Here's how the part is built. I have some questions about the finished solid (model axes, mm). A direction names the side the tool comes from. Round coordinates to 2 decimals unless told otherwise and drop trailing zeros. Write each loop counter-clockwise with the first axis right and the second up, starting at its lowest first coordinate (ties: lowest second). Pieces come first, ordered by that corner, then holes. Notation, with made-up numbers: (86, 43) -> (120, 43) arc R22 ccw to (120, 79) -> close; hole circle Ø6 at (89.25, -37). An arc over 180 degrees is marked (long way). Answer in a Markdown table with one row per item. Add a question column.
Autodesk Inventor part; units mm, degrees
ref_plane "YZ Plane" through (0, 0, 0) normal (1, 0, 0) x (0, 1, 0)
ref_plane "XZ Plane" through (0, 0, 0) normal (0, 1, 0) x (-1, 0, 0)
ref_plane "XY Plane" through (0, 0, 0) normal (0, 0, 1) x (1, 0, 0)
sketch "Sketch1" plane through (0, 0, 0) normal (0, 1, 0) x (-1, 0, 0)
  circle A0 centre (0, 0) radius 450
  circle A1 centre (0, 0) radius 470
  line L0 (470, 0) -> (450, 0)
  line L1 (-470, 0) -> (-450, 0)
  line L2 (0, 0) -> (-389.7114, 225) construction
  line L3 (0, 450) -> (0, 0) construction
  line L4 (0, 470) -> (0, 450)
  line L5 (-389.7114, 225) -> (-407.0319, 235)
  line L6 (-389.6755, 233.0622) -> (-400.0678, 239.0622)
  line L7 (-400.0678, 239.0622) -> (-401.3614, 231.7261)
  line L8 (-389.6755, 233.0622) -> (-395.382, 228.2739)
  line L9 (-398.3717, 230) -> (-394.8717, 236.0622) construction
  line L10 (7, 454) -> (0, 456.5478)
  line L11 (7, 454) -> (7, 466)
  line L12 (7, 466) -> (0, 463.4522)
  line L13 (396.6755, 220.9378) -> (395.382, 228.2739)
  line L14 (396.6755, 220.9378) -> (407.0678, 226.9378)
  line L15 (407.0678, 226.9378) -> (401.3614, 231.7261)
  line L16 (389.6755, -233.0622) -> (395.382, -228.2739)
  line L17 (389.6755, -233.0622) -> (400.0678, -239.0622)
  line L18 (400.0678, -239.0622) -> (401.3614, -231.7261)
  line L19 (-7, -454) -> (0, -456.5478)
  line L20 (-7, -454) -> (-7, -466)
  line L21 (-7, -466) -> (0, -463.4522)
  line L22 (-396.6755, -220.9378) -> (-395.382, -228.2739)
  line L23 (-396.6755, -220.9378) -> (-407.0678, -226.9378)
  line L24 (-407.0678, -226.9378) -> (-401.3614, -231.7261)
  line L25 (-363.084, 285.1192) -> (-343.7989, 308.0994)
  line L26 (-343.7989, 308.0994) -> (-341.3477, 306.0423)
  line L27 (-341.3477, 306.0423) -> (-360.6327, 283.0622)
  line L28 (-360.6327, 283.0622) -> (-363.084, 285.1192)
  line L29 (-363.084, 285.1192) -> (-341.3477, 306.0423) construction
  line L30 (-343.7989, 308.0994) -> (-360.6327, 283.0622) construction
  circle A2 centre (0, 0) radius 460.0533 construction
  line L31 (-435.6969, 142.6478) -> (-438.7038, 143.7424)
  line L32 (-438.7038, 143.7424) -> (-428.4415, 171.9326)
  line L33 (-425.4346, 170.8379) -> (-435.6969, 142.6478)
  line L34 (-428.4415, 171.9326) -> (-425.4346, 170.8379)
  line L35 (-458.2096, -14.9721) -> (-461.4096, -14.9719)
  line L36 (-461.4096, -14.9719) -> (-461.4077, 15.0281)
  line L37 (-458.2077, 15.0279) -> (-458.2096, -14.9721)
  line L38 (-461.4077, 15.0281) -> (-458.2077, 15.0279)
  line L39 (-425.4554, -170.786) -> (-428.4625, -171.8803)
  line L40 (-428.4625, -171.8803) -> (-438.7214, -143.6889)
  line L41 (-435.7143, -142.5946) -> (-425.4554, -170.786)
  line L42 (-438.7214, -143.6889) -> (-435.7143, -142.5946)
  line L43 (-341.385, -306.0007) -> (-343.8365, -308.0575)
  line L44 (-343.8365, -308.0575) -> (-363.1187, -285.075)
  line L45 (-360.6673, -283.0182) -> (-341.385, -306.0007)
  line L46 (-363.1187, -285.075) -> (-360.6673, -283.0182)
  line L47 (-216.1386, -404.3072) -> (-217.7388, -407.0783)
  line L48 (-217.7388, -407.0783) -> (-243.7186, -392.0768)
  line L49 (-242.1185, -389.3056) -> (-216.1386, -404.3072)
  line L50 (-243.7186, -392.0768) -> (-242.1185, -389.3056)
  line L51 (-64.8227, -453.8482) -> (-65.3785, -456.9996)
  line L52 (-65.3785, -456.9996) -> (-94.9224, -451.7883)
  line L53 (-94.3666, -448.637) -> (-64.8227, -453.8482)
  line L54 (-94.9224, -451.7883) -> (-94.3666, -448.637)
  line L55 (94.3118, -448.6485) -> (94.8673, -451.7999)
  line L56 (94.8673, -451.7999) -> (65.3228, -457.0075)
  line L57 (64.7673, -453.8561) -> (94.3118, -448.6485)
  line L58 (65.3228, -457.0075) -> (64.7673, -453.8561)
  line L59 (242.071, -389.3351) -> (243.6708, -392.1065)
  line L60 (243.6708, -392.1065) -> (217.6891, -407.1049)
  line L61 (216.0893, -404.3335) -> (242.071, -389.3351)
  line L62 (217.6891, -407.1049) -> (216.0893, -404.3335)
  line L63 (360.6327, -283.0622) -> (363.084, -285.1192)
  line L64 (363.084, -285.1192) -> (343.7989, -308.0994)
  line L65 (341.3477, -306.0423) -> (360.6327, -283.0622)
  line L66 (343.7989, -308.0994) -> (341.3477, -306.0423)
  line L67 (435.6969, -142.6478) -> (438.7038, -143.7424)
  line L68 (438.7038, -143.7424) -> (428.4415, -171.9326)
  line L69 (425.4346, -170.8379) -> (435.6969, -142.6478)
  line L70 (428.4415, -171.9326) -> (425.4346, -170.8379)
  line L71 (458.2096, 14.9721) -> (461.4096, 14.9719)
  line L72 (461.4096, 14.9719) -> (461.4077, -15.0281)
  line L73 (458.2077, -15.0279) -> (458.2096, 14.9721)
  line L74 (461.4077, -15.0281) -> (458.2077, -15.0279)
  line L75 (425.4554, 170.786) -> (428.4625, 171.8803)
  line L76 (428.4625, 171.8803) -> (438.7214, 143.6889)
  line L77 (435.7143, 142.5946) -> (425.4554, 170.786)
  line L78 (438.7214, 143.6889) -> (435.7143, 142.5946)
  line L79 (341.385, 306.0007) -> (343.8365, 308.0575)
  line L80 (343.8365, 308.0575) -> (363.1187, 285.075)
  line L81 (360.6673, 283.0182) -> (341.385, 306.0007)
  line L82 (363.1187, 285.075) -> (360.6673, 283.0182)
  line L83 (216.1386, 404.3072) -> (217.7388, 407.0783)
  line L84 (217.7388, 407.0783) -> (243.7186, 392.0768)
  line L85 (242.1185, 389.3056) -> (216.1386, 404.3072)
  line L86 (243.7186, 392.0768) -> (242.1185, 389.3056)
  line L87 (64.8227, 453.8482) -> (65.3785, 456.9996)
  line L88 (65.3785, 456.9996) -> (94.9224, 451.7883)
  line L89 (94.3666, 448.637) -> (64.8227, 453.8482)
  line L90 (94.9224, 451.7883) -> (94.3666, 448.637)
  line L91 (-94.3118, 448.6485) -> (-94.8673, 451.7999)
  line L92 (-94.8673, 451.7999) -> (-65.3228, 457.0075)
  line L93 (-64.7673, 453.8561) -> (-94.3118, 448.6485)
  line L94 (-65.3228, 457.0075) -> (-64.7673, 453.8561)
  line L95 (-242.071, 389.3351) -> (-243.6708, 392.1065)
  line L96 (-243.6708, 392.1065) -> (-217.6891, 407.1049)
  line L97 (-216.0893, 404.3335) -> (-242.071, 389.3351)
  line L98 (-217.6891, 407.1049) -> (-216.0893, 404.3335)
  point P0 (460, 0)
  point P1 (-460, 0)
  point P2 (7, 460)
  point P3 (401.8717, 223.9378)
  point P4 (394.8717, -236.0622)
  point P5 (-7, -460)
  point P6 (-401.8717, -223.9378)
  point P7 (-352.2158, 295.5808)
  point P8 (7, 460)
  point P9 (-361.8584, 284.0907)
  point P10 (-342.5733, 307.0709)
  point P11 (-437.2004, 143.1951)
  point P12 (-426.938, 171.3853)
  point P13 (-459.8096, -14.972)
  point P14 (-459.8077, 15.028)
  point P15 (-426.959, -171.3332)
  point P16 (-437.2178, -143.1418)
  point P17 (-342.6108, -307.0291)
  point P18 (-361.893, -284.0466)
  point P19 (-216.9387, -405.6927)
  point P20 (-242.9185, -390.6912)
  point P21 (-65.1006, -455.4239)
  point P22 (-94.6445, -450.2126)
  point P23 (94.5896, -450.2242)
  point P24 (65.045, -455.4318)
  point P25 (242.8709, -390.7208)
  point P26 (216.8892, -405.7192)
  point P27 (361.8584, -284.0907)
  point P28 (342.5733, -307.0709)
  point P29 (437.2004, -143.1951)
  point P30 (426.938, -171.3853)
  point P31 (459.8096, 14.972)
  point P32 (459.8077, -15.028)
  point P33 (426.959, 171.3332)
  point P34 (437.2178, 143.1418)
  point P35 (342.6108, 307.0291)
  point P36 (361.893, 284.0466)
  point P37 (216.9387, 405.6927)
  point P38 (242.9185, 390.6912)
  point P39 (65.1006, 455.4239)
  point P40 (94.6445, 450.2126)
  point P41 (-94.5896, 450.2242)
  point P42 (-65.045, 455.4318)
  point P43 (-242.8709, 390.7208)
  point P44 (-216.8892, 405.7192)
  dimension "d0" = 900
  dimension "d1" = 940
  dimension "d4" = 60
  dimension "d5" = 7
  dimension "d6" = 70
  dimension "d8" = 12
  dimension "d11" = 360
  dimension "d13" = 3.2
  dimension "d14" = 30
  dimension "d15" = 50
  dimension "d18" = 360
extrude "Extrusion1" add sketch "Sketch1" along normal blind 3 contours A0 L5 L8 L6 L7 A1 L4 | L4 L12 L11 L10
properties part number "D90_CM_CIRCULO"
Item 1: If we section it at D-D on x = 258: Please give me the cut outline in (y, z) (3 decimals).
Item 2: If we mould it in two halves opening along Z, with no side actions, what happens to faces 1 (the cylindrical face through (237.977, 1.479, 405.298)), 2 (the flat face through (353.576, 1.479, 296.448)), 3 (the cylindrical face through (227.85, 1.48, 388.05))? For each: pulls with the +Z half, pulls with the -Z half, needs draft (parallel to the pull), parting line crosses it, or undercut.
Item 3: I need wall thicknesses on line 1 along X through (y, z) = (0.55, 392.5); line 2 along X through (y, z) = (2.65, 289.5); line 3 along Z through (x, y) = (68, 0.5). Which ranges of each line are inside material? Lowest first, please. Write a range as from..to.
Item 4: If we section it at C-C on z = 339.5: Please give me the cut outline in (x, y).
Item 5: If we section it at B-B on y = 2.15: Please give me the cut outline in (x, z).
Item 6: On a 3-axis mill with a long thin cutter (end or side, diameter ignored), from which of +Z, -Z, +X, -X, +Y, -Y can I reach the whole of each face in a straight line? I mean faces 4 (the flat face through (230.86, 1.48, 399.5)), 5 (the flat face through (216, 3, 403)). Say none if no direction works.
Item 7: For P1, Ø1.5, axis at y = 0.5, z = 406, coming from the -X side, with a flat end and sliding along its axis, tell me the tip position at first contact or that it passes through.
Item 8: If we section it at A-A on x = 75: Please give me the cut outline in (y, z).
Results list:
| question | item | result |
|---|---|---|
| 1 | outline | (0, 368.695) -> (3, 368.695) -> (3, 392.856) -> (0, 392.856) -> close |
| 2 | face 1 | pulls with the +Z half |
| 2 | face 2 | undercut |
| 2 | face 3 | pulls with the -Z half |
| 3 | line 1 | 220.1..236.59, 242.99..258.54 |
| 3 | line 2 | 344.51..355.23, 359.41..370.26 |
| 3 | line 3 | 444.83..453.29, 456.54..465.05 |
| 4 | outline | (295.36, 0) -> (325.02, 0) -> (325.02, 3) -> (295.36, 3) -> close |
| 5 | outline | (-7, 454) -> (0, 456.55) -> (0, 450) arc R450 cw to (389.71, 225) -> (395.38, 228.27) -> (389.68, 233.06) -> (400.07, 239.06) -> (401.36, 231.73) -> (407.03, 235) arc R470 ccw to (0, 470) -> (0, 463.45) -> (-7, 466) -> close; hole (64.77, 453.86) -> (94.31, 448.65) -> (94.87, 451.8) -> (65.32, 457.01) -> close; hole (216.09, 404.33) -> (242.07, 389.34) -> (243.67, 392.11) -> (217.69, 407.1) -> close; hole (341.35, 306.04) -> (360.63, 283.06) -> (363.08, 285.12) -> (343.8, 308.1) -> close |
| 6 | face 4 | +Y, -Y |
| 6 | face 5 | +Z, -Z, +X, -X, +Y |
| 7 | P1 | x = 192.5 |
| 8 | outline | (0, 443.71) -> (3, 443.71) -> (3, 452.05) -> (0, 452.05) -> close; (0, 455.3) -> (3, 455.3) -> (3, 463.98) -> (0, 463.98) -> close |
